Design review of the part shown in the three views and the two pictorial views. Dimensions are in mm from the part's minimum x, y and z. Give positions to 0.01 mm unless a question says otherwise; leave off trailing zeros. Order: outer loops, then holes, each group sorted by start corner. A loop starts at its lowest first (then second) coordinate and runs counter-clockwise, first axis right, second up. Notation, with made-up numbers: M 14.5,28 L 23.5,28 A14 ccw 23.5,36 Z; hole C -7,22.25 d11. An arc over 180 degrees is marked long. Answer as a JSON object with one key per item and string values.
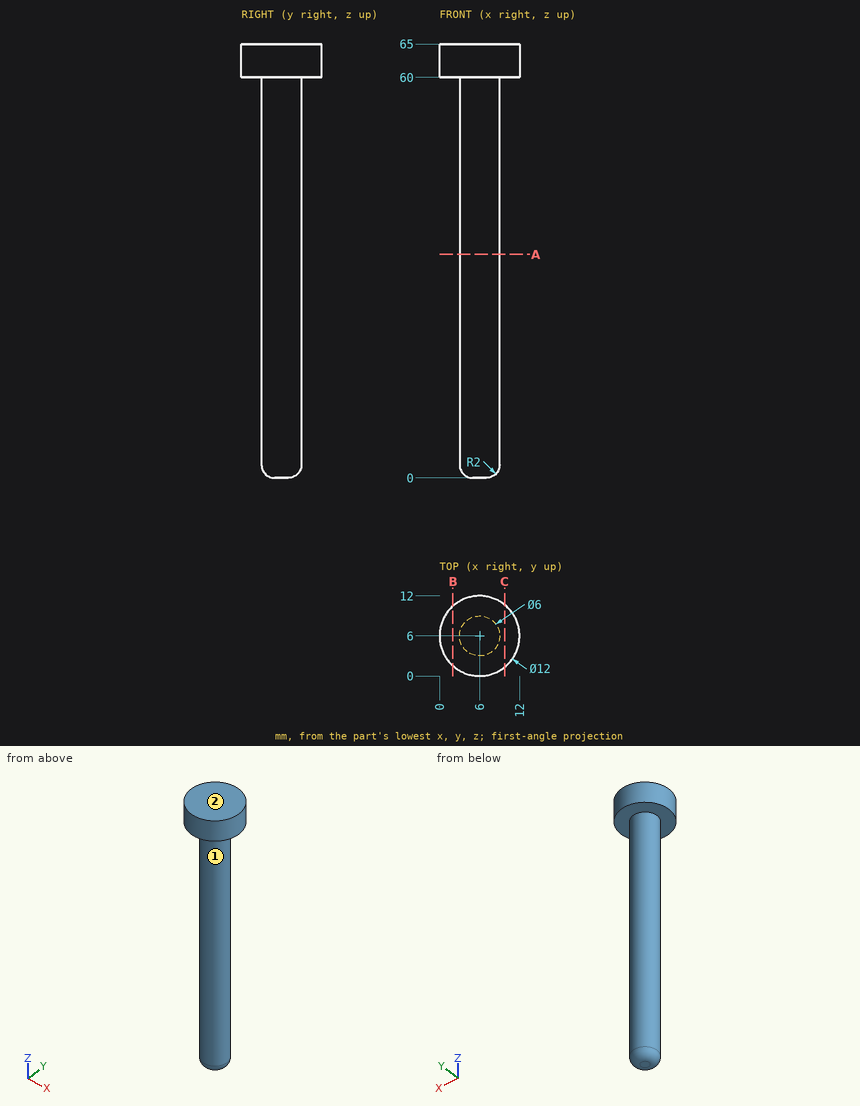
(1) We need section C-C (x = 9.75). Write out the cut boundary in (y, z).
Checked values:
{"outline": "M 1.32,60 L 10.68,60 L 10.68,65 L 1.32,65 Z"}
(2) Draft analysis for pull direction X (two halves, no side actions). For the marked faces 1 and 2, state which applies: +X half, -X half, draft (parallel to the pull), parting line (faces both ways), or undercut.
Checked values:
{"face 1": "parting line", "face 2": "draft"}
(3) To check wall thickness, follow L1, parallel to Z at x = 3.25, y = 1; L2, parallel to X at y = 6.5, z = 16.5; L3, parallel to Z at x = 7, y = 8.5. State the ranges of each line that lie inside material, in increasing order. Write a range as from..to.
Checked values:
{"L1": "z = 60..65", "L2": "x = 3.04..8.96", "L3": "z = 0.93..65"}
(4) Insertion check: pin 1 (2 mm diameter, centred on x = 5.5, z = 17, fed in from +Y); pin 2 (5 mm diameter, centred on x = 9, y = 7.5, fed in from -Z); pin 3 (5 mm diameter, centred on x = 6, z = 42, fed in from -Y); pin 4 (3 mm diameter, centred on x = 3.5, z = 20.5, fed in from -Y). Each pin has a flat end and moves straight along its axis. Give the tip position at first contact, or say it passes through.
Checked values:
{"pin 1": "stops at y = 9", "pin 2": "stops at z = 0", "pin 3": "stops at y = 3", "pin 4": "stops at y = 3.17"}
(5) We need section A-A (z = 33.5). Write out the cut boundary in (x, y), plus the area to 3 significant figures.
Checked values:
{"outline": "C 6,6 d6", "area": "28.3 mm^2"}
(6) We need section B-B (x = 2). Write out the cut boundary in (y, z).
Checked values:
{"outline": "M 1.53,60 L 10.47,60 L 10.47,65 L 1.53,65 Z"}
